from build123d import *

# Parameters (mm, degrees)
PAD_DEPTH       = 16
SKETCH014_R     = 3.25
POCKET007_DEPTH = 10
SKETCH017_R     = 3.25
POCKET008_DEPTH = 5


with BuildPart() as part:
    # Sketch → Pad (new body, symmetric)
    with BuildSketch(Plane.YZ):
        with BuildLine():
            Line((-5, 9), (-5, 41))
            ThreePointArc((4, 50), (-2.363961, 47.363961), (-5, 41))
            Line((4, 50), (36.5, 50))
            ThreePointArc((45.5, 41), (42.863961, 47.363961), (36.5, 50))
            Line((45.5, 9), (45.5, 41))
            ThreePointArc((45.5, 9), (46.671573, 6.171573), (49.5, 5))
            Line((49.5, 5), (66.25, 5))
            ThreePointArc((70.25, 1), (69.078427, 3.828427), (66.25, 5))
            Line((70.25, 0), (70.25, 1))
            Line((-29.75, 0), (70.25, 0))
            Line((-29.75, 0), (-29.75, 1))
            ThreePointArc((-25.75, 5), (-28.578427, 3.828427), (-29.75, 1))
            Line((-25.75, 5), (-9, 5))
            ThreePointArc((-9, 5), (-6.171573, 6.171573), (-5, 9))
        make_face()
        with BuildLine():
            ThreePointArc((4, 45), (1.171573, 43.828427), (0, 41))
            Line((0, 9), (0, 41))
            ThreePointArc((0, 9), (1.171573, 6.171573), (4, 5))
            Line((36.5, 5), (4, 5))
            ThreePointArc((36.5, 5), (39.328427, 6.171573), (40.5, 9))
            Line((40.5, 41), (40.5, 9))
            ThreePointArc((40.5, 41), (39.328427, 43.828427), (36.5, 45))
            Line((4, 45), (36.5, 45))
        make_face(mode=Mode.SUBTRACT)
    extrude(amount=PAD_DEPTH, both=True)

    # Sketch014 → Pocket007 (cut)
    with BuildSketch(Plane.XY.offset(50)):
        with Locations((0, 20.25)):
            Circle(SKETCH014_R)
    extrude(amount=-POCKET007_DEPTH, mode=Mode.SUBTRACT)

    # Sketch017 (on Face13 of Pocket007) → Pocket008 (cut)
    with BuildSketch(Plane(origin=(0, 0, 5), x_dir=(0, -1, 0), z_dir=(0, 0, 1))):
        with Locations((-57.75, 0)):
            Circle(SKETCH017_R)
        with Locations((17.25, 0)):
            Circle(SKETCH017_R)
    extrude(amount=-POCKET008_DEPTH, mode=Mode.SUBTRACT)


solid = part.part
Here's how the part is built. I have some questions about the finished solid (model axes, mm). A direction names the side the tool comes from. Round coordinates to 2 decimals unless told otherwise and drop trailing zeros. Order: outer loops, then holes, each group sorted by start corner. A loop starts at its lowest first (then second) coordinate and runs counter-clockwise, first axis right, second up. Notation, with made-up numbers: (26.25, 58) -> (56.25, 58) arc R28 cw to (56.25, 95) -> close; hole circle Ø1 at (38.25, -2). An arc over 180 degrees is marked (long way). Use CSV: the item, a comma, the result in double quotes.
1. Thinking about a two-plate mould opening in X: for faces 4 (the face through (0, 0, 25)), 5 (the face through (0, 61, 3)), 6 (the face through (-16, 20.5, 4.7)), which applies, pulls with the +X half, pulls with the -X half, needs draft (parallel to the pull), parting line crosses it, or undercut?
Recorded:
face 4,"needs draft"
face 5,"undercut"
face 6,"pulls with the -X half"
2. I want a section at A-A on x = 0. Give the number of separate pieces and of enclosed holes in the cut face, and give its area (3 significant figures).
Recorded:
separate pieces,"3"
enclosed holes,"0"
area,"1,030 mm2"
3. I want a section at C-C on y = 20.25. List the corners of the cut face in (x, z) for me.
Recorded:
outline,"(-16, 0) -> (16, 0) -> (16, 5) -> (-16, 5) -> close; (-16, 45) -> (-3.25, 45) -> (-3.25, 50) -> (-16, 50) -> close; (3.25, 45) -> (16, 45) -> (16, 50) -> (3.25, 50) -> close"
4. I need wall thicknesses on line 1 along Z through (x, y) = (6.5, 8.5); line 2 along Y through (x, z) = (-13, 21); line 3 along X through (y, z) = (57.75, 3.7). Which ranges of each line are inside material? Lowest first, please.
Recorded:
line 1,"z = 0 to 5, 45 to 50"
line 2,"y = -5 to 0, 40.5 to 45.5"
line 3,"x = -16 to -3.25, 3.25 to 16"
5. I want a section at B-B on z = 11. List the corners of the cut face in (x, y) for me, and give its area (3 significant figures).
Recorded:
outline,"(-16, -5) -> (16, -5) -> (16, 0) -> (-16, 0) -> close; (-16, 40.5) -> (16, 40.5) -> (16, 45.5) -> (-16, 45.5) -> close"
area,"320 mm2"
6. I'm going to push flat-ended pins straight in: P1, Ø1, axis at x = -8.5, z = 29, coming from the -Y side; P2, Ø4, axis at x = 0, y = -17.25, coming from the -Z side; P3, Ø4, axis at x = 5.5, y = 44, coming from the +Z side; P4, Ø5, axis at x = 0, y = 20.25, coming from the +Z side. Where does each tip first touch, or does it pass through?
Recorded:
P1,"stops at y = -5"
P2,"passes through"
P3,"stops at z = 48.12"
P4,"stops at z = 5"
7. Which directions (+Z, -Z, +X, -X, +Y, -Y) give clear straight access to the entire face, cutting with the end or side of a thin tool? Please do faces 1 (the face through (0.224, 39.359, 43.797)), 2 (the face through (-0.705, 17.077, 47.535)), 3 (the face through (0, -5, 25)).
Recorded:
face 1,"+X, -X"
face 2,"+Z"
face 3,"+Z, +X, -X, -Y"
8. I want a section at D-D on y = -17.25. List the corners of the cut face in (x, z) for me, and give its area (4 significant figures).
Recorded:
outline,"(-16, 0) -> (-3.25, 0) -> (-3.25, 5) -> (-16, 5) -> close; (3.25, 0) -> (16, 0) -> (16, 5) -> (3.25, 5) -> close"
area,"127.5 mm2"
